```python
from build123d import *

# Parameters (mm, degrees)
F1_DEPTH = 20
F2_R     = 9.99999
F3_R     = 4
F3_R_2   = 1.5
F4_DEPTH = 55.501


# Not quite as in the source:
# - a fillet or chamfer is up to 0.001 mm smaller than in the source, because OpenCascade refuses the exact size


with BuildPart() as f1:
    # F0 (on Top) → F1 (new body)
    with BuildSketch(Plane.XY):
        Polygon((-27.75, 37), (-27.75, 0), (-25.75, 0), (-25.75, 35), (25.75, 35), (25.75, 0), (27.75, 0), (27.75, 37), align=None)
    extrude(amount=F1_DEPTH)

    # F2 (radius 10 in the source; OpenCascade refuses exactly that, so slightly less here)
    f2_edges = [f1.edges().sort_by_distance(p)[0] for p in [
        (-26.75, 0, 0),
        (-26.75, 0, 20),
        (26.75, 0, 0),
        (26.75, 0, 20),
    ]]
    fillet(f2_edges, radius=F2_R)

    # F3 (on face) → F4 (cut, through all)
    with BuildSketch(Plane(origin=(-27.75, 0, 0), x_dir=(0, -1, 0), z_dir=(-1, 0, 0))):
        with Locations((-10, 10)):
            Circle(F3_R)
        with Locations((-10, 3)):
            Circle(F3_R_2)
        with Locations((-10, 17)):
            Circle(F3_R_2)
        with Locations((-3, 10)):
            Circle(F3_R_2)
        with Locations((-17, 10)):
            Circle(F3_R_2)
    extrude(amount=-F4_DEPTH, mode=Mode.SUBTRACT)


solid = f1.part
```
Source: CAD feature listing. Evaluate the final solid. Frame: model axes, mm. A direction names the side the tool comes from. Give positions to 0.01 mm unless a question says otherwise; leave off trailing zeros. Loops run counter-clockwise (first coordinate to the right, second up) from the corner with the lowest first, then second, coordinate; pieces in that order, holes last. Notation, with made-up numbers: M 11.5,-36 L 56.5,-36 A25 ccw 56.5,-2 Z; hole C 35.25,37.5 d10. An arc over 180 degrees is marked long. Put each result on its own line as item: value.
Q1. Pin query (flat end, axial travel): P1, Ø8, axis at x = 21.5, y = 7, coming from the +Z side; P2, Ø4, axis at x = -12.5, z = 8, coming from the -Y side. Return the tip coordinate at first contact, or that it passes through.
Response values:
P1: passes through
P2: stops at y = 35
Q2. Reachability of faces 1 (the cylindrical face through (-26.764, 1.614, 9.425)), 2 (the flat face through (25.75, 22, 10)) from +Z, -Z, +X, -X, +Y, -Y: full face, straight path, thin tool, end or side. Return the list, or none.
Response values:
face 1: +X, -X
face 2: +Z, -Z, -Y
Q3. Section A-A (y = 17). Return the cut outline in (x, z).
Response values:
outline: M -27.75,0 L -25.75,0 L -25.75,8.5 L -27.75,8.5 Z; M -27.75,11.5 L -25.75,11.5 L -25.75,20 L -27.75,20 Z; M 25.75,0 L 27.75,0 L 27.75,8.5 L 25.75,8.5 Z; M 25.75,11.5 L 27.75,11.5 L 27.75,20 L 25.75,20 Z
Q4. Line query: probe 1 along Z at (x, y) = (26.9, 10); probe 2 along X at (y, z) = (2, 8.25); probe 3 along Z at (x, y) = (26.65, 17). Output: solid intervals per line, ascending. Write a range as [from, to].
Response values:
probe 1: z = [0, 1.5], [4.5, 6], [14, 15.5], [18.5, 20]
probe 2: x = [-27.75, -25.75], [25.75, 27.75]
probe 3: z = [0, 8.5], [11.5, 20]
Q5. Section D-D (z = 16.25). Return the cut outline in (x, y).
Response values:
outline: M -27.75,2.19 L -25.75,2.19 L -25.75,8.7 L -27.75,8.7 Z; M -27.75,11.3 L -25.75,11.3 L -25.75,35 L 25.75,35 L 25.75,11.3 L 27.75,11.3 L 27.75,37 L -27.75,37 Z; M 25.75,2.19 L 27.75,2.19 L 27.75,8.7 L 25.75,8.7 Z
Q6. Mould query, pull axis Z, two halves, no side actions, for faces 3 (the flat face through (-2, 36, 20)), 4 (the flat face through (-25.75, 21, 10)), 5 (the cylindrical face through (-26.76, 18.5, 10.07)). Classes: released by +Z, released by -Z, zero draft, split by the parting line, or undercut.
Response values:
face 3: released by +Z
face 4: zero draft
face 5: undercut
Q7. Section C-C (x = 17.5). Return the cut outline in (y, z).
Response values:
outline: M 35,0 L 37,0 L 37,20 L 35,20 Z
Q8. Section B-B (z = 6.75). Return the cut outline in (x, y), and give its area (3 significant figures).
Response values:
outline: M -27.75,0.54 L -25.75,0.54 L -25.75,7.67 L -27.75,7.67 Z; M -27.75,12.33 L -25.75,12.33 L -25.75,35 L 25.75,35 L 25.75,12.33 L 27.75,12.33 L 27.75,37 L -27.75,37 Z; M 25.75,0.54 L 27.75,0.54 L 27.75,7.67 L 25.75,7.67 Z
area: 230 mm²
